Can you work these out from the model? Positions are in its coordinate system, mm. Give positions to 0.01 mm unless a question says otherwise; leave off trailing zeros. Loops run counter-clockwise (first coordinate to the right, second up) from the corner with the lowest first, then second, coordinate; pieces in that order, holes last. Notation, with made-up numbers: (-6, -25) - (33, -25) arc R23 ccw to (33, -15) - close; hole circle Ø11 at (34, -25). An arc over 180 degrees is marked (long way). Answer in a Markdown table with one row per item.
from build123d import *

# Parameters (mm, degrees)
F0_W     = 750
F0_H     = 250
F1_DEPTH = 25
F2_R     = 4
F3_DEPTH = 5
F4_R     = 2
F5_R     = 2
F7_D     = 8.8
F7_DEPTH = 12
F7_TIP   = 2.6437867237


with BuildPart() as f1:
    # F0 (on Front) → F1 (new body)
    with BuildSketch(Plane.XZ):
        Rectangle(F0_W, F0_H)
    extrude(amount=F1_DEPTH)

    # F2 (on face) → F3 (join)
    with BuildSketch(Plane(origin=(0, 0, -125), x_dir=(1, 0, 0), z_dir=(0, 0, -1))):
        with Locations((-367, 17)):
            Circle(F2_R)
        with Locations((367, 17)):
            Circle(F2_R)
    extrude(amount=F3_DEPTH)

    # F4
    f4_edges = [f1.edges().sort_by_distance(p)[0] for p in [
        (0, -25, -125),
    ]]
    fillet(f4_edges, radius=F4_R)

    # F5
    f5_edges = [f1.edges().sort_by_distance(p)[0] for p in [
        (-375, -11.5, -125),
        (375, -11.5, -125),
    ]]
    fillet(f5_edges, radius=F5_R)

    # F7
    with Locations(Plane.XZ.offset(25)):
        with Locations((-335, 80), (-295, 80), (-295, -80), (-335, -80), (295, 80), (335, 80), (295, -80), (335, -80)):
            Hole(F7_D / 2, depth=F7_DEPTH)
            with Locations((0, 0, -(F7_DEPTH + F7_TIP / 2))):  # 118° drill point
                Cone(0, F7_D / 2, F7_TIP, mode=Mode.SUBTRACT)


solid = f1.part
Q1. If we mould it in two halves opening along X, with no side actions, what happens to faces 1 (the face through (-5, -11, -125)), 2 (the face through (-5, -25, 3)), 3 (the face through (375, -11, -1))? For each: released by +X, released by -X, zero draft, split by the parting line, or undercut.
Checked values:
| item | result |
|---|---|
| face 1 | undercut |
| face 2 | zero draft |
| face 3 | released by +X |
Q2. If I drill on line 1 (Z direction, x = 295, y = -15.25); line 2 (X direction, y = -19.25, z = 80); line 3 (Z direction, x = -91.5, y = -16.75), over which ranges is the centre line in solid material (lowest first)? Write a range as [from, to].
Checked values:
| item | result |
|---|---|
| line 1 | z = [-125, -84.4], [-75.6, 75.6], [84.4, 125] |
| line 2 | x = [-375, -339.4], [-330.6, -299.4], [-290.6, 290.6], [299.4, 330.6], [339.4, 375] |
| line 3 | z = [-125, 125] |
Q3. Imagine slicing it at A-A, the plane x = -152. Write out the boundary of the cut face in (y, z), and give its area (3 significant figures).
Checked values:
| item | result |
|---|---|
| outline | (-25, -123) arc R2 ccw to (-23, -125) - (0, -125) - (0, 125) - (-25, 125) - close |
| area | 6,250 mm² |
Q4. For pin 1 (7 mm diameter, centred on x = 295, z = 80, fed in from +Y); pin 2 (3 mm diameter, centred on x = -264.5, y = -18.5, fed in from -Z); pin 3 (8 mm diameter, centred on x = -335, z = 80, fed in from -Y); pin 4 (7 mm diameter, centred on x = -335, z = -80, fed in from -Y), each with a flat end and sliding along its axis, tell me the tip position at first contact or that it passes through.
Checked values:
| item | result |
|---|---|
| pin 1 | stops at y = 0 |
| pin 2 | stops at z = -125 |
| pin 3 | stops at y = -12.76 |
| pin 4 | stops at y = -12.46 |
